Verification items for the finished model (mm, model axes). A direction names the side the tool comes from. Round coordinates to 2 decimals unless told otherwise and drop trailing zeros. Order: outer loops, then holes, each group sorted by start corner. A loop starts at its lowest first (then second) coordinate and runs counter-clockwise, first axis right, second up. Notation, with made-up numbers: (2, 74) -> (22, 74) arc R24 ccw to (22, 85) -> close; hole circle Ø4 at (50.5, -12.5). An arc over 180 degrees is marked (long way). Return JSON: item names as keys, results as strings. Group by question number.
1) Tool access check on faces 5 (the cylindrical face through (13.196, 0.07, 4.289)), 6 (the cylindrical face through (-7.454, 2.64, 0.986)), 7 (the flat face through (-9, 11, 1)), 8 (the flat face through (2.5, -8, 1)). Record the directions out of +Z, -Z, +X, -X, +Y, -Y that give a thin tool (end or side, any length) a straight path to the whole face; none if there is none.
2) Section check D-D on y = 1. Enter the section's corners in (x, z).
3) Section check A-A on y = -4.5. Enter the section's corners in (x, z), plus the area to 3 significant figures.
4) Section check B-B on x = -0.5. Enter the section's corners in (y, z), plus the area to 3 significant figures.
5) Section check C-C on z = 4. State how many separate pieces and enclosed holes the cut face has, plus the area to 3 significant figures.
6) Depth check by flat-ended pin: pin 1 (2 mm diameter, centred on x = 7, y = 11.5, fed in from +Z); pin 2 (0.6 mm diameter, centred on y = -7, z = 1.5, fed in from -X); pin 3 (1.8 mm diameter, centred on x = 8.5, y = -7.5, fed in from +Z); pin 4 (0.6 mm diameter, centred on y = 14, z = 1, fed in from -X). Enter the tip coordinate at first touch or a pass-through.
7) Draft check along Y on faces 1 (the cylindrical face through (0.07, -13.196, 4.289)), 2 (the cylindrical face through (-13.196, -0.07, 4.289)), 3 (the cylindrical face through (-0.07, 12.39, 4.95)), 4 (the cylindrical face through (-7.61, 10.31, 0.49)). Enter one of: pulls with the +Y half, pulls with the -Y half, needs draft (parallel to the pull), parting line crosses it, or undercut.
8) Scan lines: L1, parallel to Z at x = 5.5, y = 8.5; L2, parallel to X at y = -6.5, z = 0.75; L3, parallel to X at y = -7.5, z = 4. Record each from-to range of solid material in increasing order.
Solid Edge part; units mm, degrees
sketch "Sketch1" plane through (0, 0, 0) normal (0, 0, 1) x (1, 0, 0)
  line L0 (-5, 15) -> (5, 15)
  arc A0 (15, 5) -> (5, 15) centre (5, 5) ccw
  line L1 (15, 5) -> (15, -5)
  arc A1 (5, -15) -> (15, -5) centre (5, -5) ccw
  line L2 (5, -15) -> (-5, -15)
  arc A2 (-15, -5) -> (-5, -15) centre (-5, -5) ccw
  line L3 (-15, -5) -> (-15, 5)
  arc A3 (-5, 15) -> (-15, 5) centre (-5, 5) ccw
extrude "Protrusion1" add sketch "Sketch1" along normal blind 6
sketch "Sketch2" plane through (0, 0, 0) normal (0, 0, -1) x (-1, 0, 0)
  arc A0 (8, 0.5) -> (5.8943, 4.2901) centre (3.5362, 0.5) ccw
  line L0 (3.5, 15) -> (3.5356, 8.5081)
  line L1 (-3.5, 15) -> (3.5, 15)
  line L2 (-3.5, 15) -> (-3.5, 13.7321)
  line L3 (-5, 13.7321) -> (-3.5, 13.7321)
  arc A1 (-13, 8.5) -> (-5, 13.7321) centre (-5, 5) cw
  line L4 (-13, -3.5) -> (-13, 8.5)
  line L5 (-2.5, -3.5) -> (-13, -3.5)
  line L6 (-2.5, -11.5) -> (-2.5, -3.5)
  line L7 (8, -11.5) -> (-2.5, -11.5)
  line L8 (8, 0.5) -> (8, -11.5)
  arc A2 (5.8943, 4.29) -> (3.5356, 8.5081) centre (8.5355, 8.5355) cw
extrude "VaciadoExtruido_1" cut sketch "Sketch2" against normal blind 2
fillet "Redondeo_2" radius 6 7 edges at (-12.0711, -12.0711, 6) (-12.0711, 12.0711, 6) (0, 15, 6) (12.0711, 12.0711, 6) (12.0711, -12.0711, 6) (15, 0, 6) (0, -15, 6)
sketch "Sketch3" plane through (0, 0, 0) normal (0, 0, 1) x (1, 0, 0)
  circle A0 centre (-8.5355, 8.5355) radius 2
  circle A1 centre (8.5355, -8.5355) radius 2
extrude "Cutout1" cut sketch "Sketch3" along normal through all
sketch "Sketch4" plane through (0, 0, 6) normal (0, 0, 1) x (1, 0, 0)
  circle A0 centre (-8.5355, 8.5355) radius 3
  circle A1 centre (8.5355, -8.5355) radius 3
extrude "VaciadoExtruido_3" cut sketch "Sketch4" against normal blind 5
Check result:
{
 "1": {"face 5": "+Z, +X, +Y, -Y", "face 6": "-Z", "face 7": "+Z", "face 8": "-Z, +Y"},
 "2": {"outline": "(-15, 0) -> (-7.97, 0) -> (-7.97, 2) -> (13, 2) -> (13, 0) -> (15, 0) arc R6 ccw to (9, 6) -> (-9, 6) arc R6 ccw to start"},
 "3": {"outline": "(-15, 0) -> (-8, 0) -> (-8, 2) -> (2.5, 2) -> (2.5, 0) -> (15, 0) arc R6 ccw to (9, 6) -> (-9, 6) arc R6 ccw to start", "area": "144 mm^2"},
 "4": {"outline": "(-15, 0) -> (-11.5, 0) -> (-11.5, 2) -> (14.66, 2) arc R6 ccw to (9, 6) -> (-9, 6) arc R6 ccw to start", "area": "112 mm^2"},
 "5": {"separate pieces": "1", "enclosed holes": "2", "area": "608 mm^2"},
 "6": {"pin 1": "z = 5.72", "pin 2": "x = -14.7", "pin 3": "through", "pin 4": "x = -9.77"},
 "7": {"face 1": "pulls with the -Y half", "face 2": "needs draft", "face 3": "pulls with the +Y half", "face 4": "undercut"},
 "8": {"L1": "2 to 6", "L2": "-14.84 to -8, 2.5 to 14.84", "L3": "-13.09 to 5.72, 11.35 to 13.09"}
}
